Autodesk Inventor part; units mm, degrees
ref_plane "YZ Plane" through (0, 0, 0) normal (1, 0, 0) x (0, 1, 0)
ref_plane "XZ Plane" through (0, 0, 0) normal (0, 1, 0) x (-1, 0, 0)
ref_plane "XY Plane" through (0, 0, 0) normal (0, 0, 1) x (1, 0, 0)
sketch "Sketch1" plane through (0, 0, 0) normal (1, 0, 0) x (0, 1, 0)
  arc A0 (3.5, 20) -> (-3.5, 20) centre (0, 20) ccw
  line L0 (6.2139, 1.9071) -> (3.5, 20)
  line L1 (-3.5, 20) -> (-6.2139, 1.9071)
  line L2 (0, 0) -> (2.6706, 0)
  arc A1 (-3.5, -20) -> (3.5, -20) centre (0, -20) ccw
  line L3 (-3.5, -20) -> (-6.2139, -1.9071)
  line L4 (6.2139, -1.9071) -> (3.5, -20)
  arc A2 (-6.2139, 1.9071) -> (-6.2139, -1.9071) centre (0, 0) ccw
  arc A3 (6.2139, -1.9071) -> (6.2139, 1.9071) centre (0, 0) ccw
  line L5 (0, 0) -> (2.6706, 0)
  point P0 (6.5, 0)
  point P1 (-6.5, 0)
  dimension "d0" = 7
  dimension "d1" = 20
extrude "Extrusion1" add sketch "Sketch1" along normal blind 5
sketch "Sketch2" plane through (5, 0, 0) normal (1, 0, 0) x (0, 0, -1)
  line L0 (0, 6.5) -> (0.5, 6.5)
  line L1 (0.5, 6.5) -> (1.2768, 4.8342)
  line L2 (-0.5, 6.5) -> (-1.2768, 4.8342)
  line L3 (0, 6.5) -> (-0.5, 6.5)
  line L4 (-3.5142, 5.4681) -> (-3.0935, 5.7385)
  line L5 (-3.0935, 5.7385) -> (-1.5395, 4.7571)
  line L6 (-3.9348, 5.1978) -> (-3.6877, 3.3766)
  line L7 (-3.5142, 5.4681) -> (-3.9348, 5.1978)
  line L8 (-5.9126, 2.7002) -> (-5.7049, 3.155)
  line L9 (-5.7049, 3.155) -> (-3.867, 3.1696)
  line L10 (-6.1203, 2.2454) -> (-4.9278, 0.8468)
  line L11 (-5.9126, 2.7002) -> (-6.1203, 2.2454)
  line L12 (-6.4338, -0.925) -> (-6.505, -0.4301)
  line L13 (-6.505, -0.4301) -> (-4.9667, 0.5758)
  line L14 (-6.3627, -1.42) -> (-4.6033, -1.9517)
  line L15 (-6.4338, -0.925) -> (-6.3627, -1.42)
  line L16 (-4.9124, -4.2566) -> (-5.2398, -3.8787)
  line L17 (-5.2398, -3.8787) -> (-4.4896, -2.2008)
  line L18 (-4.5849, -4.6345) -> (-2.8174, -4.1307)
  line L19 (-4.9124, -4.2566) -> (-4.5849, -4.6345)
  line L20 (-1.8313, -6.2367) -> (-2.311, -6.0958)
  line L21 (-2.311, -6.0958) -> (-2.587, -4.2787)
  line L22 (-1.3515, -6.3776) -> (-0.1369, -4.9981)
  line L23 (-1.8313, -6.2367) -> (-1.3515, -6.3776)
  line L24 (1.8313, -6.2367) -> (1.3515, -6.3776)
  line L25 (1.3515, -6.3776) -> (0.1369, -4.9981)
  line L26 (2.311, -6.0958) -> (2.587, -4.2787)
  line L27 (1.8313, -6.2367) -> (2.311, -6.0958)
  line L28 (4.9124, -4.2566) -> (4.5849, -4.6345)
  line L29 (4.5849, -4.6345) -> (2.8174, -4.1307)
  line L30 (5.2398, -3.8787) -> (4.4896, -2.2008)
  line L31 (4.9124, -4.2566) -> (5.2398, -3.8787)
  line L32 (6.4338, -0.925) -> (6.3627, -1.42)
  line L33 (6.3627, -1.42) -> (4.6033, -1.9517)
  line L34 (6.505, -0.4301) -> (4.9667, 0.5758)
  line L35 (6.4338, -0.925) -> (6.505, -0.4301)
  line L36 (5.9126, 2.7002) -> (6.1203, 2.2454)
  line L37 (6.1203, 2.2454) -> (4.9278, 0.8468)
  line L38 (5.7049, 3.155) -> (3.867, 3.1696)
  line L39 (5.9126, 2.7002) -> (5.7049, 3.155)
  line L40 (3.5142, 5.4681) -> (3.9348, 5.1978)
  line L41 (3.9348, 5.1978) -> (3.6877, 3.3766)
  line L42 (3.0935, 5.7385) -> (1.5395, 4.7571)
  line L43 (3.5142, 5.4681) -> (3.0935, 5.7385)
  arc A0 (-1.2768, 4.8342) -> (-1.5395, 4.7571) centre (0, 0) ccw
  arc A1 (1.5395, 4.7571) -> (1.2768, 4.8342) centre (0, 0) ccw
  arc A2 (3.867, 3.1696) -> (3.6877, 3.3766) centre (0, 0) ccw
  arc A3 (4.9667, 0.5758) -> (4.9278, 0.8468) centre (0, 0) ccw
  arc A4 (4.4896, -2.2008) -> (4.6033, -1.9517) centre (0, 0) ccw
  arc A5 (2.587, -4.2787) -> (2.8174, -4.1307) centre (0, 0) ccw
  arc A6 (-0.1369, -4.9981) -> (0.1369, -4.9981) centre (0, 0) ccw
  arc A7 (-2.8174, -4.1307) -> (-2.587, -4.2787) centre (0, 0) ccw
  arc A8 (-4.6033, -1.9517) -> (-4.4896, -2.2008) centre (0, 0) ccw
  arc A9 (-3.6877, 3.3766) -> (-3.867, 3.1696) centre (0, 0) ccw
  arc A10 (-4.9278, 0.8468) -> (-4.9667, 0.5758) centre (0, 0) ccw
  circle A11 centre (0, 0) radius 2.5
  arc A12 (-1.9071, -6.2139) -> (1.9071, -6.2139) centre (0, 0) ccw
  line L44 (-2.311, -6.0958) -> (-2.3021, -6.1547)
  line L45 (-20, -3.5) -> (-1.9071, -6.2139)
  line L46 (-2.3021, -6.1547) -> (-1.9071, -6.2139)
  line L47 (2.311, -6.0958) -> (2.3021, -6.1547)
  line L48 (1.9071, -6.2139) -> (20, -3.5)
  line L49 (2.3021, -6.1547) -> (1.9088, -6.2139)
  arc A13 (-6.4865, -0.4181) -> (-6.4338, -0.925) centre (0, 0) ccw
  arc A14 (-5.2308, -3.8586) -> (-4.9124, -4.2566) centre (0, 0) ccw
  arc A15 (-2.3143, -6.074) -> (-1.3369, -6.361) centre (0, 0) ccw
  arc A16 (0, -6.5) -> (2.3143, -6.074) centre (0, 0) ccw
  point P0 (0, 5)
  point P1 (-2.7032, 4.2063)
  point P2 (-4.5482, 2.0771)
  point P3 (-4.9491, -0.7116)
  point P4 (-3.7787, -3.2743)
  point P5 (-1.4087, -4.7975)
  point P6 (1.4087, -4.7975)
  point P7 (3.7787, -3.2743)
  point P8 (4.9491, -0.7116)
  point P9 (4.5482, 2.0771)
  point P10 (2.7032, 4.2063)
  dimension "d8" = 0.5
  dimension "d9" = 115
  dimension "d10" = 6.5
  dimension "d11" = 360
  dimension "d12" = 5
extrude "Extrusion2" cut sketch "Sketch2" against normal blind 2.5 contours L0 L1 A1 L42 L43 L40 L41 A2 L38 L39 L36 L37 A3 L34 L35 L32 L33 A4 L30 L31 L28 L29 A5 L26 A16 L27 A12 L25 A6 L22 L20 A15 L21 A7 L18 L19 A14 L17 A8 L14 L15 A13 L13 A10 L10 L11 L8 L9 A9 L6 L7 L4 L5 A0 L2 L3 | L26 L27 A16 | A15 L20 L21 | L47 L48 L27 | L20 L45 L44 | A12 L22 A6 L25
properties part number "servo horn"
For this review, take the finished solid that the model builds, in its own axes (mm). A direction names the side the tool comes from. Round coordinates to 2 decimals unless told otherwise and drop trailing zeros. Loops run counter-clockwise (first coordinate to the right, second up) from the corner with the lowest first, then second, coordinate; pieces in that order, holes last.
Q1. Mouldability with a two-part tool opening along Y and no side actions: class faces 3 (the face through (1.2, -6.5, 0)), 4 (the face through (3.768, -4.386, 3.714)), 5 (the face through (2.465, 4.876, 10.827)) as +Y half, -Y half, draft (parallel to the pull), parting line (faces both ways), or undercut.
Result sheet:
face 3: -Y half
face 4: undercut
face 5: +Y half
Q2. To check wall thickness, follow line 1 along Z through (x, y) = (3.3, 2); line 2 along Y through (x, z) = (0.2, 10.5); line 3 along Z through (x, y) = (4.8, -2.75). State the ranges of each line that lie inside material, in increasing order.
Result sheet:
line 1: z = -22.87 to -5.91, -1.5 to 1.5, 5.91 to 22.87
line 2: y = -4.92 to 4.92
line 3: z = -22.17 to -4.74, 4.74 to 22.17
Q3. Add section B-B on z = 0. Write out the cut boundary in (x, y), plus the area to 3 significant figures.
Result sheet:
outline: (0, -6.5) - (2.5, -6.5) - (2.5, -2.5) - (5, -2.5) - (5, 2.5) - (2.5, 2.5) - (2.5, 6.5) - (0, 6.5) - close
area: 45.0 mm2
Q4. Machinability: for faces 1 (the face through (1.9, 6.5, 0)), 2 (the face through (3.768, 4.3, 3.813)), which of the approach directions +Z, -Z, +X, -X, +Y, -Y give a long, thin tool a straight path to every point of the face, cutting with its end or side? Answer none if there is none.
Result sheet:
face 1: +X, -X, +Y
face 2: +X
Q5. Add section A-A on x = 1.1. Write out the cut boundary in (y, z), plus the area to 3 significant figures.
Result sheet:
outline: (-6.21, -1.91) - (-3.5, -20) arc R3.5 ccw to (3.5, -20) - (6.21, -1.91) arc R6.5 ccw to (6.21, 1.91) - (3.5, 20) arc R3.5 ccw to (-3.5, 20) - (-6.21, 1.91) arc R6.5 ccw to start
area: 439 mm2
Q6. Add section C-C on y = 0. Write out the cut boundary in (x, z).
Result sheet:
outline: (0, -23.5) - (5, -23.5) - (5, -5.85) - (2.5, -5.85) - (2.5, -2.5) - (5, -2.5) - (5, 2.5) - (2.5, 2.5) - (2.5, 5.85) - (5, 5.85) - (5, 23.5) - (0, 23.5) - close
Q7. Insertion check: pin 1 Ø6 at (y, z) = (2.5, -12) entering from -X; pin 2 Ø1.5 at (x, z) = (4, 5.5) entering from +Y. Each pin has a flat end and moves straight along its axis. Give the tip position at first contact, or say it passes through.
Result sheet:
pin 1: stops at x = 0
pin 2: stops at y = 5.79
Q8. Add section D-D on z = 17. Write out the cut boundary in (x, y).
Result sheet:
outline: (0, -3.95) - (5, -3.95) - (5, 3.95) - (0, 3.95) - close
